The figure shows three views and two pictorial views of one solid part (mm, origin at its lowest corner). Answer the questions. Round coordinates to 2 decimals unless told otherwise and drop trailing zeros. Order: outer loops, then holes, each group sorted by start corner. A loop starts at its lowest first (then second) coordinate and runs counter-clockwise, first axis right, second up. Notation, with made-up numbers: (-38.5, 80.25) -> (-3.5, 80.25) arc R3 ccw to (-3.5, 84.25) -> close; hole circle Ø8 at (-29, 55.5). An arc over 180 degrees is marked (long way). One line per item, written item: value. Start each with the question number.
1. Section C-C (y = 7) is taken. Give the vertices of the cut face in (x, z), then the cut area to 3 significant figures.
2. Flat-ended cylindrical pins translate along their axes: pin 1 Ø1 at (y, z) = (1.5, 18) entering from -X; pin 2 Ø1.5 at (y, z) = (5, 18.5) entering from +X. Find the tip coordinate at first contact, or state that the pin passes through.
3. Section A-A (x = 6.5) is taken. Give the vertices of the cut face in (y, z).
4. Consider line 1 (Y direction, x = 19.5, z = 25); line 2 (X direction, y = 7.25, z = 6); line 3 (X direction, y = 8.5, z = 13) (1 decimal). Determine where each line is inside the solid, lowest interval first.
5. Section D-D (x = 2) is taken. Give the vertices of the cut face in (y, z), then the cut area to 3 significant figures.
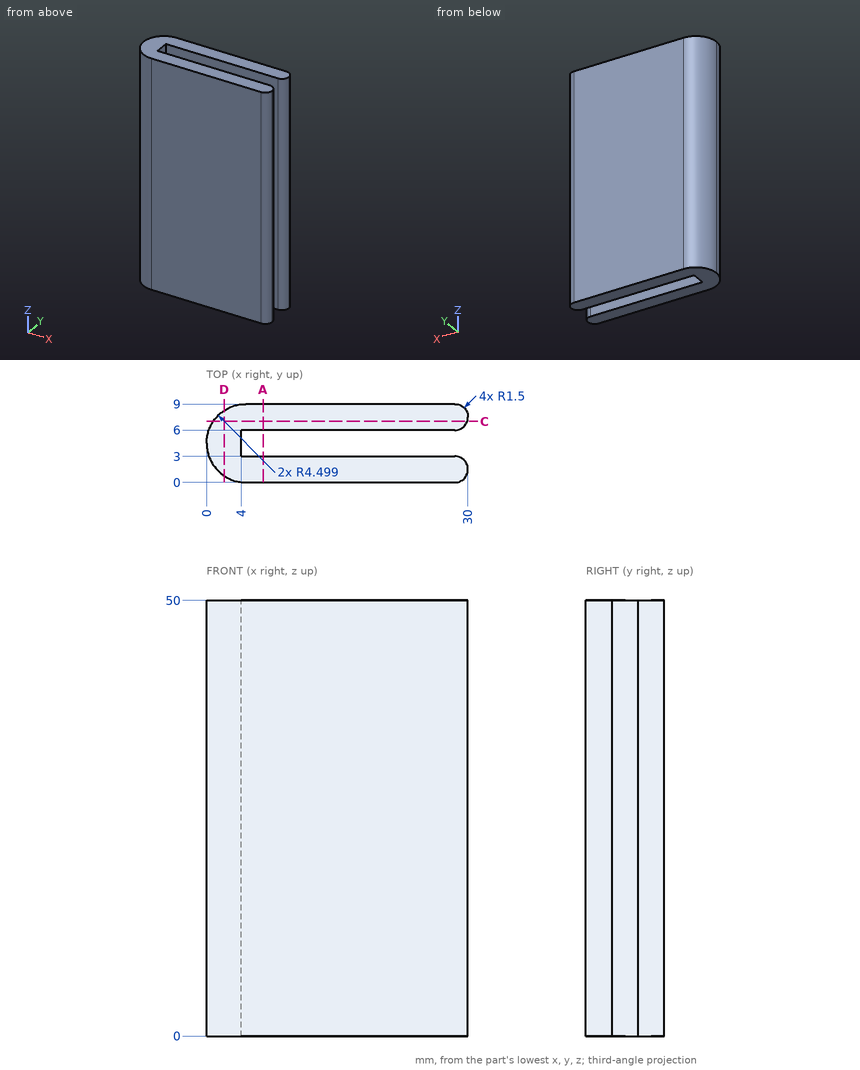
Answer:
1. outline: (0.76, 0) -> (29.91, 0) -> (29.91, 50) -> (0.76, 50) -> close
1. area: 1,460 mm^2
2. pin 1: x = 0.76
2. pin 2: x = 4
3. outline: (0, 0) -> (3, 0) -> (3, 50) -> (0, 50) -> close; (6, 0) -> (9, 0) -> (9, 50) -> (6, 50) -> close
4. line 1: 0 to 3, 6 to 9
4. line 2: 0.94 to 29.98
4. line 3: 2.4 to 29.6
5. outline: (0.76, 0) -> (8.24, 0) -> (8.24, 50) -> (0.76, 50) -> close
5. area: 374 mm^2
